from build123d import *

# Parameters (mm, degrees)
BOSS_EXTRUDE1_DEPTH  = 3.175
M3_CLEARANCE_HOLE2_D = 3.4
FILLET1_R            = 1.27


with BuildPart() as part:
    # Sketch1 → Boss-Extrude1 (new body)
    with BuildSketch(Plane(origin=(0, 0, 0), x_dir=(1, 0, 0), z_dir=(0, 1, 0))):
        Polygon((0, 0), (50.8, 0), (50.8, 5.08), (60.96, 5.08), (60.96, 15.24), (-10.16, 15.24), (-10.16, 5.08), (0, 5.08), align=None)
    extrude(amount=BOSS_EXTRUDE1_DEPTH)

    # M3 Clearance Hole2 (through all)
    with Locations(Plane(origin=(0, 3.175, 0), x_dir=(1, 0, 0), z_dir=(0, 1, 0))):
        with Locations((-3.81, 10.16), (10.3505, 5.08), (40.4495, 5.08), (54.61, 10.16)):
            Hole(M3_CLEARANCE_HOLE2_D / 2)

    # Fillet1
    fillet1_edges = [part.edges().sort_by_distance(p)[0] for p in [
        (0, 1.5875, -5.08),
        (-10.16, 1.5875, -5.08),
        (-10.16, 1.5875, -15.24),
        (60.96, 1.5875, -15.24),
        (60.96, 1.5875, -5.08),
        (50.8, 1.5875, -5.08),
        (50.8, 1.5875, 0),
        (0, 1.5875, 0),
    ]]
    fillet(fillet1_edges, radius=FILLET1_R)


solid = part.part
The model under review builds one solid part; all positions refer to its coordinate system, in mm. A direction names the side the tool comes from. Give positions to 0.01 mm unless a question says otherwise; leave off trailing zeros. Order: outer loops, then holes, each group sorted by start corner. A loop starts at its lowest first (then second) coordinate and runs counter-clockwise, first axis right, second up. Notation, with made-up numbers: M 62,-20.5 L 105,-20.5 A32 ccw 105,11.5 Z; hole C 27.25,48.5 d5. An arc over 180 degrees is marked long. Answer in a Markdown table with one row per item. Add a question column.
1. Add section A-A on x = 54.61. State the section outline as (y, z) points (3 decimals), plus the area to 3 significant figures.
2. To check wall thickness, follow line 1 along X through (y, z) = (2.5, -10.16); line 2 along Z through (x, y) = (40.5, 2.15); line 3 along Z through (x, y) = (54.61, 2.1). State the ranges of each line that lie inside material, in increasing order.
3. Add section D-D on x = 10. State the section outline as (y, z) points (3 decimals).
4. Machinability: for faces 4 (the flat face through (25, 0, -8)), 5 (the flat face through (0, 2, -3)), 6 (the flat face through (50.8, 2, -3)), which of the approach directions +Z, -Z, +X, -X, +Y, -Y give a long, thin tool a straight path to every point of the face, cutting with its end or side? Answer none if there is none.
5. Add section B-B on y = 1.85. State the section outline as (x, z) points.
6. For pin 1 Ø1.6 at (x, y) = (54, 1.5) entering from +Z, flat-tipped, find the tip position at first contact; note if it passes through.
7. Add section C-C on z = -9.5. State the section outline as (x, y) points (3 decimals).
8. Mouldability with a two-part tool opening along Z and no side actions: class faces 1 (the cylindrical face through (-4.59, 1.57, -8.65)), 2 (the flat face through (25, 3.175, -8)), 3 (the cylindrical face through (60.598, 1.61, -14.858)) as released by +Z, released by -Z, zero draft, split by the parting line, or undercut.
The answers:
| question | item | result |
|---|---|---|
| 1 | outline | M 0,-15.24 L 3.175,-15.24 L 3.175,-11.86 L 0,-11.86 Z; M 0,-8.46 L 3.175,-8.46 L 3.175,-5.08 L 0,-5.08 Z |
| 1 | area | 21.5 mm2 |
| 2 | line 1 | -10.16 to -5.51, -2.11 to 52.91, 56.31 to 60.96 |
| 2 | line 2 | -15.24 to -6.78, -3.38 to 0 |
| 2 | line 3 | -15.24 to -11.86, -8.46 to -5.08 |
| 3 | outline | M 0,-15.24 L 3.175,-15.24 L 3.175,-6.743 L 0,-6.743 Z; M 0,-3.417 L 3.175,-3.417 L 3.175,0 L 0,0 Z |
| 4 | face 4 | +Z, -Z, +X, -X, -Y |
| 4 | face 5 | +Z, -X, +Y, -Y |
| 4 | face 6 | +Z, +X, +Y, -Y |
| 5 | outline | M -10.16,-13.97 A1.27 ccw -8.89,-15.24 L 59.69,-15.24 A1.27 ccw 60.96,-13.97 L 60.96,-6.35 A1.27 ccw 59.69,-5.08 L 52.07,-5.08 A1.27 cw 50.8,-3.81 L 50.8,-1.27 A1.27 ccw 49.53,0 L 1.27,0 A1.27 ccw 0,-1.27 L 0,-3.81 A1.27 cw -1.27,-5.08 L -8.89,-5.08 A1.27 ccw -10.16,-6.35 Z; hole C -3.81,-10.16 d3.4; hole C 10.35,-5.08 d3.4; hole C 40.45,-5.08 d3.4; hole C 54.61,-10.16 d3.4 |
| 6 | pin 1 | z = -5.08 |
| 7 | outline | M -10.16,0 L -5.377,0 L -5.377,3.175 L -10.16,3.175 Z; M -2.243,0 L 53.043,0 L 53.043,3.175 L -2.243,3.175 Z; M 56.177,0 L 60.96,0 L 60.96,3.175 L 56.177,3.175 Z |
| 8 | face 1 | undercut |
| 8 | face 2 | zero draft |
| 8 | face 3 | released by -Z |
